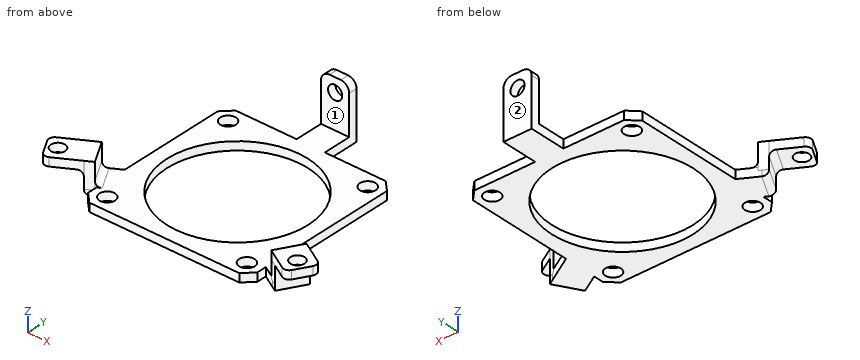
```python
from build123d import *

# Parameters (mm, degrees)
SKETCH1_R           = 2.75
SKETCH1_R_2         = 25
SKETCH1_W           = 10
SKETCH1_H           = 11
SKETCH1_H_2         = 2
BOSS_EXTRUDE1_DEPTH = 2
SKETCH5_W           = 10
SKETCH5_H           = 3
BOSS_EXTRUDE2_DEPTH = 9.1
BOSS_EXTRUDE5_DEPTH = 3
SKETCH5_2_W         = 10
SKETCH5_2_H         = 3
BOSS_EXTRUDE6_DEPTH = 18
SKETCH7_R           = 2.5
CUT_EXTRUDE1_DEPTH  = 10
SKETCH1_4_R         = 2.75
SKETCH1_4_R_2       = 25
BOSS_EXTRUDE7_DEPTH = 3
SKETCH1_5_W         = 10
SKETCH1_5_H         = 11
BOSS_EXTRUDE8_DEPTH = 3
FILLET5_R           = 2
SKETCH10_R          = 2.5
CUT_EXTRUDE2_DEPTH  = 4
FILLET6_R           = 3
FILLET7_START       = -5
FILLET7_DEPTH       = 10
FILLET7_2_DEPTH     = 10


with BuildPart() as part:
    # Sketch1 → Boss-Extrude1 (new body)
    # profile 1 of 7: a face of its own
    with BuildSketch(Plane.XY):
        Polygon((26.568542495, 30), (-26.568542495, 30), (-30, 26.568542495), (-30, -26.568542495), (-26.568542495, -30), (26.568542495, -30), (30, -26.568542495), (30, 26.568542495), align=None)
        with Locations((-24.748737342, -24.748737342)):
            Circle(SKETCH1_R, mode=Mode.SUBTRACT)
        with Locations((24.748737342, -24.748737342)):
            Circle(SKETCH1_R, mode=Mode.SUBTRACT)
        with Locations((24.748737342, 24.748737342)):
            Circle(SKETCH1_R, mode=Mode.SUBTRACT)
        with Locations((-24.748737342, 24.748737342)):
            Circle(SKETCH1_R, mode=Mode.SUBTRACT)
        Circle(SKETCH1_R_2, mode=Mode.SUBTRACT)
    # profile 2 of 7: a face of its own
    with BuildSketch(Plane.XY):
        Polygon((-30, -23.094010768), (-30, -11.547005384), (-36.267949192, -15.165807537), (-31.267949192, -23.826061575), align=None)
    # profile 3 of 7: a face of its own
    with BuildSketch(Plane.XY):
        with Locations((0, 35.5)):
            Rectangle(SKETCH1_W, SKETCH1_H)
    # profile 4 of 7: a face of its own
    with BuildSketch(Plane.XY):
        Polygon((39.739092363, -17.169872981), (30, -11.547005384), (30, -23.094010768), (34.739092363, -25.830127019), align=None)
    # profile 5 of 7: a face of its own
    with BuildSketch(Plane.XY):
        Polygon((41.47114317, -18.169872981), (39.739092363, -17.169872981), (34.739092363, -25.830127019), (36.47114317, -26.830127019), align=None)
    # profile 6 of 7: a face of its own
    with BuildSketch(Plane.XY):
        with Locations((0, 42)):
            Rectangle(SKETCH1_W, SKETCH1_H_2)
    # profile 7 of 7: a face of its own
    with BuildSketch(Plane.XY):
        Polygon((-31.267949192, -23.826061575), (-36.267949192, -15.165807537), (-38, -16.165807537), (-33, -24.826061575), align=None)
    extrude(amount=BOSS_EXTRUDE1_DEPTH)

    # Sketch5 → Boss-Extrude2 (add)
    with BuildSketch(Plane.XY.offset(2)):
        with Locations((0, 41.5)):
            Rectangle(SKETCH5_W, SKETCH5_H)
        Polygon((-38, -16.165807537), (-35.401923789, -14.665807537), (-30.401923789, -23.326061575), (-33, -24.826061575), align=None)
        Polygon((41.47114317, -18.169872981), (38.873066959, -16.669872981), (33.873066959, -25.330127019), (36.47114317, -26.830127019), align=None)
    extrude(amount=BOSS_EXTRUDE2_DEPTH)

    # Sketch6 → Boss-Extrude5 (add)
    with BuildSketch(Plane.XY.offset(11.1)):
        with BuildLine():
            Line((-46.185292351, -20.891588279), (-35.401923789, -14.665807537))
            Line((-35.401923789, -14.665807537), (-30.401923789, -23.326061575))
            Line((-30.401923789, -23.326061575), (-41.185292351, -29.551842317))
            ThreePointArc((-41.185292351, -29.551842317), (-42.739686509, -29.75648219), (-43.983511401, -28.802061782))
            Line((-43.983511401, -28.802061782), (-46.935072886, -23.68980733))
            ThreePointArc((-46.935072886, -23.68980733), (-47.139712759, -22.135413172), (-46.185292351, -20.891588279))
        make_face()
        with BuildLine():
            Line((38.897920412, -16.684222129), (33.873066959, -25.330127019))
            Line((33.873066959, -25.330127019), (41.664082648, -29.84192454))
            ThreePointArc((41.664082648, -29.84192454), (43.179952831, -30.044118571), (44.395530273, -29.116155036))
            Line((44.395530273, -29.116155036), (47.391974814, -23.960387856))
            ThreePointArc((47.391974814, -23.960387856), (47.600320032, -22.403746576), (46.645140907, -21.157081967))
            Line((46.645140907, -21.157081967), (38.897920412, -16.684222129))
        make_face()
    extrude(amount=-BOSS_EXTRUDE5_DEPTH)

    # Sketch5<2> → Boss-Extrude6 (add)
    with BuildSketch(Plane.XY.offset(2)):
        with Locations((0, 41.5)):
            Rectangle(SKETCH5_2_W, SKETCH5_2_H)
    extrude(amount=BOSS_EXTRUDE6_DEPTH)

    # Sketch7 → Cut-Extrude1 (cut)
    with BuildSketch(Plane(origin=(0, 43, 0), x_dir=(1, 0, 0), z_dir=(0, 1, 0))):
        with Locations(Location((0, -15.1, 0), (0, 0, 270))):
            Circle(SKETCH7_R)
    extrude(amount=-CUT_EXTRUDE1_DEPTH, mode=Mode.SUBTRACT)

    # Sketch1<4> → Boss-Extrude7 (add)
    with BuildSketch(Plane.XY):
        Polygon((26.568542495, 30), (-26.568542495, 30), (-30, 26.568542495), (-30, -26.568542495), (-26.568542495, -30), (26.568542495, -30), (30, -26.568542495), (30, 26.568542495), align=None)
        with Locations((-24.748737342, -24.748737342)):
            Circle(SKETCH1_4_R, mode=Mode.SUBTRACT)
        with Locations((24.748737342, -24.748737342)):
            Circle(SKETCH1_4_R, mode=Mode.SUBTRACT)
        with Locations((24.748737342, 24.748737342)):
            Circle(SKETCH1_4_R, mode=Mode.SUBTRACT)
        with Locations((-24.748737342, 24.748737342)):
            Circle(SKETCH1_4_R, mode=Mode.SUBTRACT)
        Circle(SKETCH1_4_R_2, mode=Mode.SUBTRACT)
    extrude(amount=BOSS_EXTRUDE7_DEPTH)

    # Sketch1<5> → Boss-Extrude8 (add)
    with BuildSketch(Plane.XY):
        with Locations((0, 35.5)):
            Rectangle(SKETCH1_5_W, SKETCH1_5_H)
        Polygon((-30, -23.094010768), (-30, -11.547005384), (-36.267949192, -15.165807537), (-31.267949192, -23.826061575), align=None)
        Polygon((39.739092363, -17.169872981), (30, -11.547005384), (30, -23.094010768), (34.739092363, -25.830127019), align=None)
    extrude(amount=BOSS_EXTRUDE8_DEPTH)

    # Fillet5
    fillet5_edges = [part.edges().sort_by_distance(p)[0] for p in [
        (-35.5, -20.495934556, 8.1),
    ]]
    fillet(fillet5_edges, radius=FILLET5_R)

    # Sketch10 → Cut-Extrude2 (cut)
    with BuildSketch(Plane.XY.offset(11.1)):
        with Locations((42.435244785, -24.5)):
            Circle(SKETCH10_R)
        with Locations((-42.435244785, -24.5)):
            Circle(SKETCH10_R)
    extrude(amount=-CUT_EXTRUDE2_DEPTH, mode=Mode.SUBTRACT)

    # Fillet6
    fillet6_edges = [part.edges().sort_by_distance(p)[0] for p in [
        (-5, 41.5, 20),
        (5, 41.5, 20),
    ]]
    fillet(fillet6_edges, radius=FILLET6_R)

    # Fillet7: read off the stored shape, not the designer's step
    # Fillet7 outline → Fillet7 (cut)
    with BuildSketch(Plane(origin=(0, 0, 0), x_dir=(0.8660254037844398, 0.499999999999998, 0), z_dir=(0.49999999999999795, -0.8660254037844399, 0)).offset(FILLET7_START)):
        with BuildLine():
            ThreePointArc((-38.991869112, 0), (-40.406082675, 0.585786438), (-40.991869112, 2))
            Line((-40.991869112, 2), (-40.991869112, 0))
            Line((-40.991869112, 0), (-38.991869112, 0))
        make_face()
    extrude(amount=FILLET7_DEPTH, mode=Mode.SUBTRACT)

    # Fillet7 2 outline → Fillet7 2 (add)
    with BuildSketch(Plane(origin=(0, 0, 0), x_dir=(0.8660254037844398, 0.499999999999998, 0), z_dir=(0.49999999999999795, -0.8660254037844399, 0)).offset(FILLET7_START)):
        with BuildLine():
            Line((-37.991869112, 3), (-35.991869112, 3))
            ThreePointArc((-35.991869112, 3), (-37.406082675, 3.585786438), (-37.991869112, 5))
            Line((-37.991869112, 5), (-37.991869112, 3))
        make_face()
    extrude(amount=FILLET7_2_DEPTH)


solid = part.part
```
Could you check a few things on this model? Use its own coordinates, in mm. Face numbers are marked on the shaded views. A direction names the side the tool comes from. Round coordinates to 2 decimals unless told otherwise and drop trailing zeros. Loops run counter-clockwise (first coordinate to the right, second up) from the corner with the lowest first, then second, coordinate; pieces in that order, holes last. Notation, with made-up numbers: (48, -3) - (106, -3) arc R14 ccw to (106, 12) - close; hole circle Ø4 at (49, -22). An arc over 180 degrees is marked (long way). Answer in a Markdown table with one row per item. Add a question column.
(1) If we section it at B-B (z = 15.1): Please give me the cut outline in (x, y), plus the area to 3 significant figures.
(2) If we section it at C-C (y = 0): Please give me the cut outline in (x, z), plus the area to 3 significant figures.
(3) If we section it at D-D (x = 31): Please give me the cut outline in (y, z).
(4) For the marked faces 1 and 2, which set-ups out of +Z, -Z, +X, -X, +Y, -Y let a thin tool reach every point of the face, with its end or its side?
(5) If we section it at A-A (x = 0): Please give me the cut outline in (y, z).
(6) I need wall thicknesses on line 1 along X through (y, z) = (42.3, 15.1); line 2 along Y through (x, z) = (0, 1.5); line 3 along Z through (x, y) = (37, -25.5). Which ranges of each line are inside material? Lowest first, please.
(7) I'm going to push flat-ended pins straight in: pin 1 (1 mm diameter, centred on x = 30, y = -17, fed in from +Z); pin 2 (2.5 mm diameter, centred on x = 7.5, z = 2, fed in from -Y); pin 3 (12 mm diameter, centred on x = -31.5, z = 11.5, fed in from +Y). Where does each tip first touch, or does it pass through?
Model answer:
| question | item | result |
|---|---|---|
| 1 | outline | (-5, 40) - (-2.5, 40) - (-2.5, 43) - (-5, 43) - close; (2.5, 40) - (5, 40) - (5, 43) - (2.5, 43) - close |
| 1 | area | 15.0 mm² |
| 2 | outline | (-30, 0) - (-25, 0) - (-25, 3) - (-30, 3) - close; (25, 0) - (30, 0) - (30, 3) - (25, 3) - close |
| 2 | area | 30.0 mm² |
| 3 | outline | (-23.67, 0) - (-12.12, 0) - (-12.12, 3) - (-23.67, 3) - close |
| 4 | face 1 | +Z, +X, -X, -Y |
| 4 | face 2 | +Z, -Z, +X, -X, +Y |
| 5 | outline | (-30, 0) - (-25, 0) - (-25, 3) - (-30, 3) - close; (25, 0) - (43, 0) - (43, 12.6) - (40, 12.6) - (40, 3) - (25, 3) - close; (40, 17.6) - (43, 17.6) - (43, 20) - (40, 20) - close |
| 6 | line 1 | x = -5 to -2.5, 2.5 to 5 |
| 6 | line 2 | y = -30 to -25, 25 to 43 |
| 6 | line 3 | z = 0 to 11.1 |
| 7 | pin 1 | stops at z = 3 |
| 7 | pin 2 | stops at y = -30 |
| 7 | pin 3 | stops at y = -14.67 |
